Input: dimensioned drawing with shaded views. Units: mm. Origin: part minimum x, y, z. Round coordinates to 2 decimals unless told otherwise and drop trailing zeros. Loops run counter-clockwise (first coordinate to the right, second up) from the corner with the lowest first, then second, coordinate; pieces in that order, holes last. Notation, with made-up numbers: M 16,51.5 L 40,51.5 A11 ccw 40,61.5 Z; hole C 26.25,11 d7. An arc over 180 degrees is marked long. Use one line per item in the form item = value. Start each with the question number.
Q1. Section query D-D, the plane x = 23.5. Output: boundary loops of the cut face in (y, z).
Q2. Section query C-C, the plane x = 17.5. Output: boundary loops of the cut face in (y, z) (1 decimal).
Q3. Ray query, line 1 along X through (y, z) = (3.2, 27) (1 decimal); line 2 along X through (y, z) = (1.55, 9) (1 decimal); line 3 along Y through (x, z) = (27, 25.5). Return the intervals inside material, ascending.
Q4. Section query B-B, the plane z = 32. Output: boundary loops of the cut face in (x, y) (1 decimal).
Q5. Mould query, pull axis X, two halves, no side actions, for the marked faces 1 and 2. Classes: pulls with the +X half, pulls with the -X half, needs draft (parallel to the pull), parting line crosses it, or undercut.
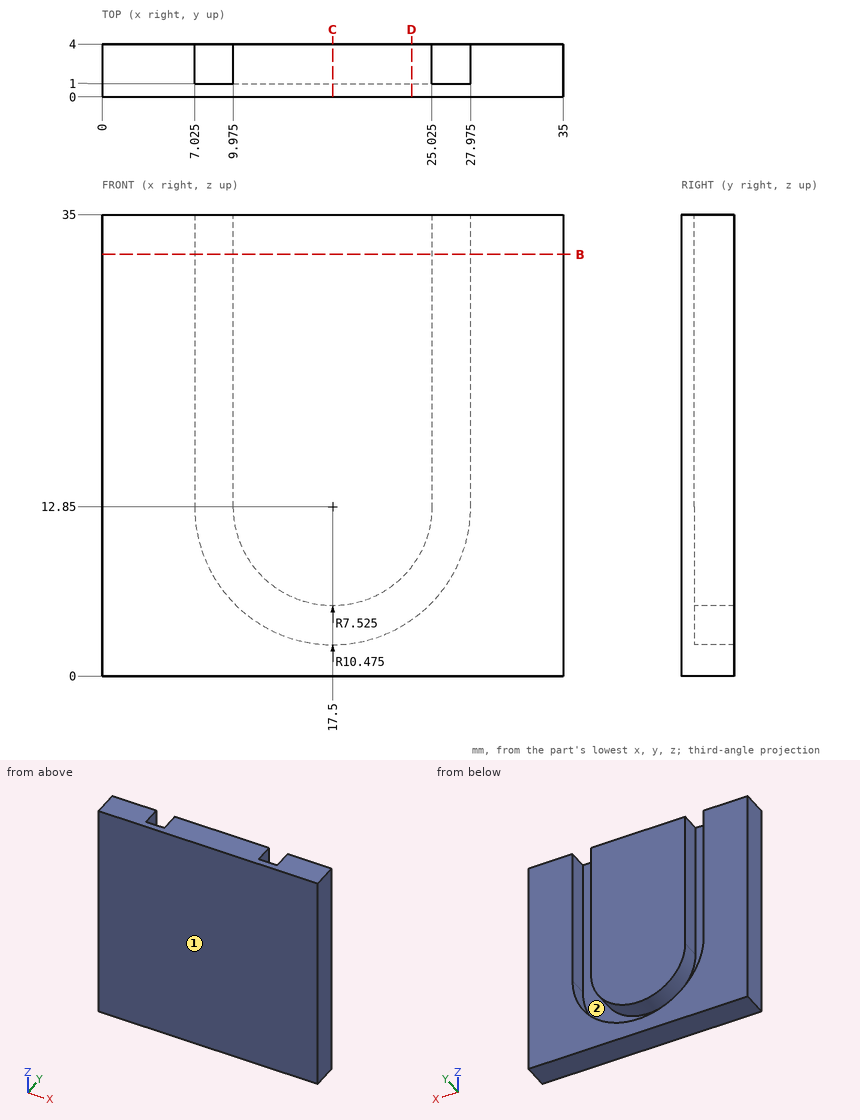
Results found:
q1.outline = M 0,0 L 4,0 L 4,4.26 L 1,4.26 L 1,8.31 L 4,8.31 L 4,35 L 0,35 Z
q2.outline = M 0,0 L 4,0 L 4,2.4 L 1,2.4 L 1,5.3 L 4,5.3 L 4,35 L 0,35 Z
q3.line_1 = 0 to 7, 10 to 25, 28 to 35
q3.line_2 = 0 to 7.8, 11 to 24, 27.2 to 35
q3.line_3 = 0 to 1
q4.outline = M 0,0 L 35,0 L 35,4 L 28,4 L 28,1 L 25,1 L 25,4 L 10,4 L 10,1 L 7,1 L 7,4 L 0,4 Z
q5.face_1 = needs draft
q5.face_2 = undercut
